Autodesk Inventor part; units mm, degrees
ref_plane "Work Plane1" through (1.525, 0, 0) normal (0, 0, 1) x (1, 0, 0)
ref_plane "YZ Plane" through (0, 0, 0) normal (1, 0, 0) x (0, 1, 0)
ref_plane "XZ Plane" through (0, 0, 0) normal (0, 1, 0) x (-1, 0, 0)
sketch "Sketch1" plane through (0, 0, 0) normal (0, 0, 1) x (1, 0, 0)
  line L0 (0, 4) -> (0, 2.5)
  line L1 (2.4, 2.5) -> (16, 2.5)
  line L2 (16, 2.5) -> (16, 0)
  line L3 (16, 0) -> (-0.5001, 0)
  line L4 (-3.8001, 0) -> (19.3, 0)
  line L5 (-0.5001, 0) -> (-0.5001, 4)
  line L6 (-0.5001, 4) -> (0, 4)
  line L7 (2.4, 2.5) -> (1.9091, 2.5)
  line L8 (1.9091, 2.5) -> (0, 2.5)
  line L9 (0, -0.8) -> (0, 4.8)
  dimension "d0" = 16
  dimension "d1" = 13.6
  dimension "d2" = 5
  dimension "d9" = 0.5001
  dimension "d10" = 8
  dimension "d13" = 0.4909
  dimension "d14" = 5
revolve "Body" add sketch "Sketch1" angle 360 about axis through (16, 0, 0) along (-1, 0, 0)
sketch "Sketch2" plane through (-0.5001, 0, 0) normal (-1, 0, 0) x (0, 0, 1)
  line L0 (0, 4.6188) -> (4, 2.3094)
  line L1 (4, 2.3094) -> (4, -2.3094)
  line L2 (4, -2.3094) -> (0, -4.6188)
  line L3 (0, -4.6188) -> (-4, -2.3094)
  line L4 (-4, -2.3094) -> (-4, 2.3094)
  line L5 (-4, 2.3094) -> (0, 4.6188)
  point P0 (0, 0)
  point P1 (0, 0)
  dimension "d11" = 8
extrude "Head" add sketch "Sketch2" along normal blind 3
sketch "Sketch4" plane through (0, 0, 0) normal (0, 0, 1) x (1, 0, 0)
  line L0 (-3.5001, 4) -> (-3.5001, 4.6188)
  line L1 (-3.5001, 4.6188) -> (-3.1428, 4.6188)
  line L2 (-3.1428, 4.6188) -> (-3.5001, 4)
  line L3 (-4.1001, 0) -> (0.0999, 0)
  line L4 (-0.5001, 4.6188) -> (-3.5001, 4.6188)
  line L5 (-3.5001, 2.3094) -> (-3.5001, 4.6188)
  dimension "d5" = 30
  dimension "d19" = 8
revolve "Chamfer1" cut sketch "Sketch4" angle 360 about axis through (-10, 0, 0) along (1, 0, 0)
thread "Thread"
chamfer "Chamfer2" distance 0.4908 distance2 0.4909 1 edges at (16, -2.5, 0) measured on face at (16, 0.6587, 0.3326)
ref_plane "Work Plane1" through (1.525, 0, 0) normal (0, 0, 1) x (1, 0, 0)
equation "\"d0\" = NLG"
equation "\"d1\" = GEL"
equation "\"d2\" = GD"
equation "\"d10\" = SD2"
equation "\"d14\" = BDM"
equation "\"d11\" = SW"
equation "\"d3\" = KOH - SD"
equation "\"d5\" = ANG1"
equation "\"d19\" = SW0"
equation "\"d15\" = GEL"
equation "\"d6\" = -0.5 * SPD + 0.5 * GD"
equation "\"NLG\" = 16"
equation "\"GD\" = NND"
equation "\"BDM\" = NND"
equation "\"KOH\" = 3.5"
equation "\"GEL\" = 13.6"
equation "\"SW\" = 8"
equation "\"SW0\" = SW"
equation "\"SPD\" = NND - 1.2269 * PTC"
equation "\"SD2\" = SW"
equation "\"SD\" = 0.5"
equation "\"ANG1\" = 30deg"
equation "\"GAL\" = 0.61345 * PTC"
equation "\"GUL\" = 0.61345 * PTC"
equation "\"RR\" = 0.2"
equation "\"WFT\" = SD"
equation "\"GD1\" = THREADDIA - 1.2269 * PTC"
equation "\"THREADDIA\" = 5"
equation "\"SDH\" = SW"
equation "\"TOA\" = 30deg"
equation "\"FAWI\" = 45deg"
equation "\"PTC\" = 0.8"
equation "\"NND\" = 5"
equation "\"E0\" = 1.155 * SW"
properties part number "AS 1110 - M5 x 16" material "Steel, Mild"
Build history of the part. All positions in model axes, mm. A direction names the side the tool comes from. Coordinates: 2 decimals unless noted, no trailing zeros. Order: outer loops, then holes, each group sorted by start corner. A loop starts at its lowest first (then second) coordinate and runs counter-clockwise, first axis right, second up. Notation, with made-up numbers: (24.25, 69) - (48.25, 69) arc R20 ccw to (48.25, 94) - close; hole circle Ø10 at (-28.75, 38). An arc over 180 degrees is marked (long way). Write item = value, one per line. Start each with the question number.
1) Saw through at B-B on x = 1.25. Write the cut outline in (y, z), then the cut area to 3 significant figures.
2) Wall check: line 1 along X through (y, z) = (3.25, -0.25); line 2 along Y through (x, z) = (7.25, -1.5). Give the ranges that are in metal, low to high. Write a range as from..to.
3) 3-axis set-ups, long thin cutter, end or side, ignore diameter. For faces 4 (the face through (7.86, -0.54, -2.44)), 5 (the face through (-0.5, -2.1, 3.6)), 6 (the face through (-0.5, 2.1, -3.6)): which of +Z, -Z, +X, -X, +Y, -Y reach the whole face in a straight line?
4) Two-plate mould, pull along X, no slides. Class faces 1 (the face through (-2, 0, -4)), 2 (the face through (-3.41, 2.07, -3.6)), 3 (the face through (-0.5, 4.2, 0)): pulls with the +X half, pulls with the -X half, needs draft (parallel to the pull), parting line crosses it, or undercut.
5) Flat gauge pins, fed straight in: pin 1 Ø1 at (x, z) = (10.5, 2.5) entering from -Y; pin 2 Ø1.3 at (y, z) = (4.5, -0.5) entering from +X; pin 3 Ø1.6 at (y, z) = (1, -3) entering from +X. Where does each tip first touch, or does it go through?
6) Saw through at A-A on x = -1.5. Write the cut outline in (y, z).
From the geometry:
q1.outline = circle Ø5 at (0, 0)
q1.area = 19.6 mm^2
q2.line_1 = -3.5..0
q2.line_2 = -2..2
q3.face_4 = +X
q3.face_5 = +Z, +X, -Y
q3.face_6 = -Z, +X, +Y
q4.face_1 = needs draft
q4.face_2 = pulls with the -X half
q4.face_3 = pulls with the +X half
q5.pin_1 = -1.5
q5.pin_2 = 0
q5.pin_3 = 15.65
q6.outline = (-4.62, 0) - (-2.31, -4) - (2.31, -4) - (4.62, 0) - (2.31, 4) - (-2.31, 4) - close
